The listing builds one solid part. Answer for the finished solid, in the listing's coordinates (mm). A direction names the side the tool comes from. Give positions to 0.01 mm unless a question says otherwise; leave off trailing zeros. Write each loop counter-clockwise with the first axis right and the second up, starting at its lowest first coordinate (ties: lowest second). Pieces come first, ordered by that corner, then holes. Notation, with made-up numbers: (46.5, 81) - (73.5, 81) arc R24 cw to (73.5, 115) - close; hole circle Ø3 at (38.25, 44). An arc over 180 degrees is marked (long way). Write each question's results on one line, items separated by ' | '. Start each with the question number.
Q1. For a pull along X with two mould halves and no side action, classify faces 6 (the face through (25, 1.5, -26)), 7 (the face through (1.5, 2, -52)), 8 (the face through (2.95, 0.76, -61.07)) as pulls with the +X half, pulls with the -X half, needs draft (parallel to the pull), parting line crosses it, or undercut.
Q2. Section B-B (x = 2.5) is taken. Determine the outline of the cut face in (y, z).
Q3. Section C-C (x = 21) is taken. Determine the outline of the cut face in (y, z).
Q4. Section D-D (z = -54) is taken. Determine the outline of the cut face in (x, y), plus the area to 3 significant figures.
Q5. Flat-ended cylindrical pins translate along their axes: pin 1 Ø0.6 at (y, z) = (3, -52) entering from -X; pin 2 Ø4 at (x, z) = (47.5, -62.5) entering from +Y; pin 3 Ø2 at (x, y) = (14, 3) entering from -Z. Find the tip coordinate at first contact, or state that the pin passes through.
Q6. For faces 1 (the face through (45, 2, -52)), 2 (the face through (25, 1, 0)), 3 (the face through (23, 2, -46)), 4 (the face through (23, 2, -58)), 5 (the face through (50, 1, -32)), determine the directions among +Z, -Z, +X, -X, +Y, -Y from which every point of the face is accessible in a straight line to the end or side of a thin tool.
Q7. Find the intervals of material crossed by probe 1 along X at (y, z) = (1.1, -62.5); probe 2 along Z at (x, y) = (36.5, 2.9); probe 3 along Y at (x, z) = (28, -45), in increasing order.
Q8. Section A-A (z = -62.5) is taken. Determine the outline of the cut face in (x, y).
```python
from build123d import *

# Parameters (mm, degrees)
SKETCH1_W           = 50
SKETCH1_H           = 44
SKETCH1_H_2         = 21
BOSS_EXTRUDE1_DEPTH = 1.5
SKETCH2_W           = 43.5
SKETCH2_H           = 12
BOSS_EXTRUDE3_DEPTH = 2
SKETCH4_R           = 1.5
CUT_EXTRUDE1_DEPTH  = 1.5


with BuildPart() as part:
    # Sketch1 → Boss-Extrude1 (new body)
    with BuildSketch(Plane(origin=(0, 0, 0), x_dir=(1, 0, 0), z_dir=(0, 1, 0))):
        with Locations((25, 22)):
            Rectangle(SKETCH1_W, SKETCH1_H)
        with Locations((25, 54.5)):
            Rectangle(SKETCH1_W, SKETCH1_H_2)
    extrude(amount=BOSS_EXTRUDE1_DEPTH)

    # Sketch2 → Boss-Extrude3 (add)
    with BuildSketch(Plane(origin=(0, 1.5, 0), x_dir=(1, 0, 0), z_dir=(0, 1, 0))):
        with Locations((23.25, 52)):
            Rectangle(SKETCH2_W, SKETCH2_H)
    extrude(amount=BOSS_EXTRUDE3_DEPTH)

    # Sketch4 → Cut-Extrude1 (cut)
    with BuildSketch(Plane(origin=(0, 1.5, 0), x_dir=(1, 0, 0), z_dir=(0, 1, 0))):
        with Locations(Location((2.5, 62.5, 0), (0, 0, 270))):
            Circle(SKETCH4_R)
        with Locations(Location((47.5, 62.5, 0), (0, 0, 270))):
            Circle(SKETCH4_R)
    extrude(amount=-CUT_EXTRUDE1_DEPTH, mode=Mode.SUBTRACT)


solid = part.part
```
Answers below:
1) face 6: needs draft | face 7: pulls with the -X half | face 8: undercut
2) outline: (0, -65) - (1.5, -65) - (1.5, -64) - (0, -64) - close; (0, -61) - (1.5, -61) - (1.5, -58) - (3.5, -58) - (3.5, -46) - (1.5, -46) - (1.5, 0) - (0, 0) - close
3) outline: (0, -65) - (1.5, -65) - (1.5, -58) - (3.5, -58) - (3.5, -46) - (1.5, -46) - (1.5, 0) - (0, 0) - close
4) outline: (0, 0) - (50, 0) - (50, 1.5) - (45, 1.5) - (45, 3.5) - (1.5, 3.5) - (1.5, 1.5) - (0, 1.5) - close | area: 162 mm2
5) pin 1: stops at x = 1.5 | pin 2: stops at y = 1.5 | pin 3: stops at z = -58
6) face 1: +Z, -Z, +X, +Y | face 2: +Z, +X, -X, +Y, -Y | face 3: +Z, +X, -X, +Y | face 4: -Z, +X, -X, +Y | face 5: +Z, -Z, +X, +Y, -Y
7) probe 1: x = 0 to 1, 4 to 46, 49 to 50 | probe 2: z = -58 to -46 | probe 3: y = 0 to 1.5
8) outline: (0, 0) - (1, 0) - (1, 1.5) - (0, 1.5) - close; (4, 0) - (46, 0) - (46, 1.5) - (4, 1.5) - close; (49, 0) - (50, 0) - (50, 1.5) - (49, 1.5) - close
